Check sheet for the modelled part. Datum: model origin and axes. Units: mm. Coordinates: 2 decimals unless noted, no trailing zeros. Loops run counter-clockwise (first coordinate to the right, second up) from the corner with the lowest first, then second, coordinate; pieces in that order, holes last. Notation, with made-up numbers: M 12,82.25 L 67,82.25 A24 cw 67,101.25 Z; hole C 60.25,22.5 d10. An arc over 180 degrees is marked long. Answer as CSV lines item,"result". Start each with the question number.
from build123d import *
from OCP.BRepAlgoAPI import BRepAlgoAPI_Cut
from OCP.TopTools import TopTools_ListOfShape

# Parameters (mm, degrees)
SISTEMA_START              = -170.205087805
SISTEMA_ESTRUCTURAL2_DEPTH = 250
CORTAR_EXTRUIR2_DEPTH      = 32


with BuildPart() as part:
    # Sistema estructural2: read off the stored shape, not the designer's step
    # Sistema estructural2 outline → Sistema estructural2 (new body)
    with BuildSketch(Plane.XY.offset(SISTEMA_START)):
        with BuildLine():
            ThreePointArc((15, 9.8), (13.476955262, 13.476955262), (9.8, 15))
            Line((9.8, 15), (-9.8, 15))
            ThreePointArc((-9.8, 15), (-13.476955262, 13.476955262), (-15, 9.8))
            Line((-15, 9.8), (-15, -9.8))
            ThreePointArc((-15, -9.8), (-13.476955262, -13.476955262), (-9.8, -15))
            Line((-9.8, -15), (9.8, -15))
            ThreePointArc((9.8, -15), (13.476955262, -13.476955262), (15, -9.8))
            Line((15, -9.8), (15, 9.8))
        make_face()
        with BuildLine():
            ThreePointArc((12.4, -9.8), (11.638477631, -11.638477631), (9.8, -12.4))
            Line((9.8, -12.4), (-9.8, -12.4))
            ThreePointArc((-9.8, -12.4), (-11.638477631, -11.638477631), (-12.4, -9.8))
            Line((-12.4, -9.8), (-12.4, 9.8))
            ThreePointArc((-12.4, 9.8), (-11.638477631, 11.638477631), (-9.8, 12.4))
            Line((-9.8, 12.4), (9.8, 12.4))
            ThreePointArc((9.8, 12.4), (11.638477631, 11.638477631), (12.4, 9.8))
            Line((12.4, 9.8), (12.4, -9.8))
        make_face(mode=Mode.SUBTRACT)
    extrude(amount=SISTEMA_ESTRUCTURAL2_DEPTH)


with BuildPart() as cortar_extruir2_tool:
    # Croquis10 → Cortar-Extruir2 (new body)
    with BuildSketch(Plane(origin=(0, 15, 0), x_dir=(1, 0, 0), z_dir=(0, 1, 0))):
        with BuildLine():
            Line((-15, -79.794912195), (15, -79.794912195))
            ThreePointArc((15, -79.794912195), (0, -64.794912195), (-15, -79.794912195))
        make_face()
        with BuildLine():
            Line((-15, 170.205087805), (15, 170.205087805))
            ThreePointArc((15, 170.205087805), (0, 155.205087805), (-15, 170.205087805))
        make_face()
    extrude(amount=-CORTAR_EXTRUIR2_DEPTH)


with BuildPart() as part_1:
    add(part.part)

    # Cortar-Extruir2: cut by cortar_extruir2_tool, with a tolerance
    cortar_extruir2_stock = TopTools_ListOfShape()
    cortar_extruir2_stock.Append(part_1.part.wrapped)
    cortar_extruir2_tools = TopTools_ListOfShape()
    cortar_extruir2_tools.Append(cortar_extruir2_tool.part.wrapped)
    cortar_extruir2_cut = BRepAlgoAPI_Cut()
    cortar_extruir2_cut.SetArguments(cortar_extruir2_stock)
    cortar_extruir2_cut.SetTools(cortar_extruir2_tools)
    cortar_extruir2_cut.SetFuzzyValue(0.00001)
    cortar_extruir2_cut.Build()
    add(Compound.cast(cortar_extruir2_cut.Shape()).solids(), mode=Mode.REPLACE)


solid = part_1.part
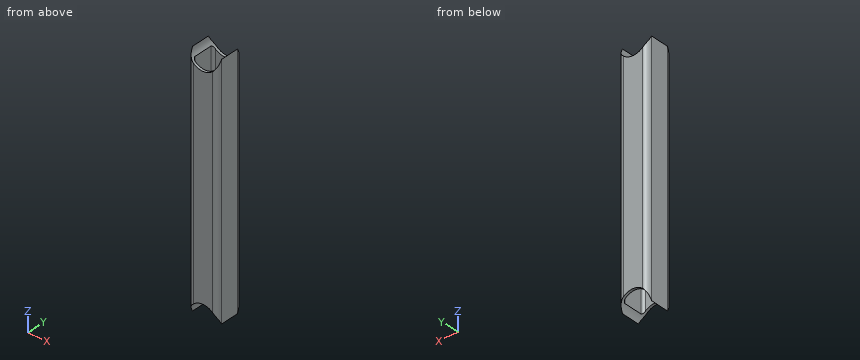
Item 1: Material ranges on line 1 (X direction, y = -2, z = 7.5); line 2 (Y direction, x = -12, z = 51), recorded low to high. Write a range as from..to.
Item 2: Sectioned sample at C-C, the plane z = -96. Record the boundary of the cut face in (x, y), and give its area (3 significant figures).
Item 3: Sectioned sample at B-B, the plane y = 2.5. Record the boundary of the cut face in (x, z).
Item 4: Go/stop test with a flat-tipped pin: pin 1 (3 mm diameter, centred on x = -11, z = -87, fed in from -Y). Record where the tip stops, or that it passes through.
Item 5: Sectioned sample at A-A, the plane x = 0. Record the boundary of the cut face in (y, z), and give its area (3 significant figures).
Reply:
1,line 1,"-15..-12.4, 12.4..15"
1,line 2,"-14.51..-11.19, 11.19..14.51"
2,outline,"M -15,-9.8 A5.2 ccw -9.8,-15 L 9.8,-15 A5.2 ccw 15,-9.8 L 15,9.8 A5.2 ccw 9.8,15 L -9.8,15 A5.2 ccw -15,9.8 Z; hole M -12.4,-9.8 A2.6 ccw -9.8,-12.4 L 9.8,-12.4 A2.6 ccw 12.4,-9.8 L 12.4,9.8 A2.6 ccw 9.8,12.4 L -9.8,12.4 A2.6 ccw -12.4,9.8 Z"
2,area,"268 mm²"
3,outline,"M -15,-170.21 A15 cw -12.4,-161.76 L -12.4,71.35 A15 cw -15,79.79 Z; M 12.4,-161.76 A15 cw 15,-170.21 L 15,79.79 A15 cw 12.4,71.35 Z"
4,pin 1,"y = -15"
5,outline,"M -15,-155.21 L -12.4,-155.21 L -12.4,64.79 L -15,64.79 Z; M 12.4,-155.21 L 15,-155.21 L 15,64.79 L 12.4,64.79 Z"
5,area,"1,140 mm²"
